from build123d import *

# Parameters (mm, degrees)
SKETCH1_W           = 60
SKETCH1_H           = 70
SKETCH1_R           = 18
BOSS_EXTRUDE1_DEPTH = 10
FILLET1_R           = 2
SKETCH3_R           = 4.5
CUT_EXTRUDE2_DEPTH  = 100


with BuildPart() as part:
    # Sketch1 → Boss-Extrude1 (new body)
    with BuildSketch(Plane.XY):
        Rectangle(SKETCH1_W, SKETCH1_H)
        Circle(SKETCH1_R, mode=Mode.SUBTRACT)
    extrude(amount=BOSS_EXTRUDE1_DEPTH)

    # Fillet1
    fillet1_edges = [part.edges().sort_by_distance(p)[0] for p in [
        (-30, -35, 5),
        (-30, 35, 5),
        (30, 35, 5),
        (30, -35, 5),
    ]]
    fillet(fillet1_edges, radius=FILLET1_R)

    # Sketch3 → Cut-Extrude2 (cut)
    with BuildSketch(Plane(origin=(-387.472155748, 43.575337974, 11), x_dir=(-1, 0, 0), z_dir=(0, 0, -1))):
        with Locations(Location((-407.472155748, -68.575337974, 0), (0, 0, 180))):
            Circle(SKETCH3_R)
        with Locations(Location((-367.472155748, -68.575337974, 0), (0, 0, 180))):
            Circle(SKETCH3_R)
        with Locations(Location((-367.472155748, -18.575337974, 0), (0, 0, 180))):
            Circle(SKETCH3_R)
        with Locations(Location((-407.472155748, -18.575337974, 0), (0, 0, 180))):
            Circle(SKETCH3_R)
    extrude(amount=CUT_EXTRUDE2_DEPTH, mode=Mode.SUBTRACT)


solid = part.part
The model under review builds one solid part; all positions refer to its coordinate system, in mm. Round coordinates to 2 decimals unless told otherwise and drop trailing zeros. Loops run counter-clockwise (first coordinate to the right, second up) from the corner with the lowest first, then second, coordinate; pieces in that order, holes last. Notation, with made-up numbers: M 54.5,4.5 L 86.5,4.5 A20 cw 86.5,17.5 Z; hole C 31.25,72 d6. An arc over 180 degrees is marked long. Answer as CSV lines item,"result". Start each with the question number.
Item 1: Consider section D-D (y = 0). Write out the cut boundary in (x, z), then the cut area to 3 significant figures.
Item 2: Consider section C-C (x = 0). Write out the cut boundary in (y, z), then the cut area to 3 significant figures.
Item 3: Insertion check: P1, Ø1.5, axis at x = -18, y = 15.5, coming from the -Z side; P2, Ø5.5, axis at x = -20, y = 25, coming from the +Z side. Each pin has a flat end and moves straight along its axis. Give the tip position at first contact, or say it passes through.
Item 4: Wall thickness on line 1 (Y direction, x = -20, z = 5.25); line 2 (Y direction, x = 22, z = 9); line 3 (Y direction, x = 0, z = 6.5): over which ranges is each line inside the solid? List them lowest first. Write a range as [from, to].
Item 5: Consider section A-A (x = -20). Write out the cut boundary in (y, z), then the cut area to 3 significant figures.
Item 6: Mouldability with a two-part tool opening along X and no side actions: class faces 1 (the face through (-29.43, -34.4, 5.07)), 2 (the face through (-23.32, 21.96, 5.07)), 3 (the face through (0, 35, 5)) as released by +X, released by -X, zero draft, split by the parting line, or undercut.
Item 7: Consider section B-B (y = -25). Write out the cut boundary in (x, z), then the cut area to 3 significant figures.
Answer:
1,outline,"M -30,0 L -18,0 L -18,10 L -30,10 Z; M 18,0 L 30,0 L 30,10 L 18,10 Z"
1,area,"240 mm^2"
2,outline,"M -35,0 L -18,0 L -18,10 L -35,10 Z; M 18,0 L 35,0 L 35,10 L 18,10 Z"
2,area,"340 mm^2"
3,P1,"stops at z = 0"
3,P2,"passes through"
4,line 1,"y = [-35, -29.5], [-20.5, 20.5], [29.5, 35]"
4,line 2,"y = [-35, -29.03], [-20.97, 20.97], [29.03, 35]"
4,line 3,"y = [-35, -18], [18, 35]"
5,outline,"M -35,0 L -29.5,0 L -29.5,10 L -35,10 Z; M -20.5,0 L 20.5,0 L 20.5,10 L -20.5,10 Z; M 29.5,0 L 35,0 L 35,10 L 29.5,10 Z"
5,area,"520 mm^2"
6,face 1,"released by -X"
6,face 2,"undercut"
6,face 3,"zero draft"
7,outline,"M -30,0 L -24.5,0 L -24.5,10 L -30,10 Z; M -15.5,0 L 15.5,0 L 15.5,10 L -15.5,10 Z; M 24.5,0 L 30,0 L 30,10 L 24.5,10 Z"
7,area,"420 mm^2"
